```python
from build123d import *

# Parameters (mm, degrees)
CHANFREIN1_SIZE                                = 0.2
FRAISAGE_POUR_VIS_T_TE_FRAIS_E_M31_D           = 3.4
FRAISAGE_POUR_VIS_T_TE_FRAIS_E_M31_CSINK_D     = 6.3
FRAISAGE_POUR_VIS_T_TE_FRAIS_E_M31_CSINK_ANGLE = 90
CONG_1_R                                       = 2
FRAISAGE_POUR_VIS_T_TE_FRAIS_E_M22_D           = 2.2
FRAISAGE_POUR_VIS_T_TE_FRAIS_E_M22_CSINK_D     = 4.4
FRAISAGE_POUR_VIS_T_TE_FRAIS_E_M22_CSINK_ANGLE = 90


with BuildPart() as part:
    # Esquisse1 → Révolution1 (revolve)
    with BuildSketch(Plane(origin=(0, 0, 0), x_dir=(0, 0, -1), z_dir=(1, 0, 0))):
        Polygon((-5, -3), (-5, 0), (-8.5, 0), (-8.5, 6), (-18, 6), (-18, 3), (-11, 3), (-11, -3), align=None)
    revolve(axis=Axis((0, 0, 0), (0, -1, 0)))

    # Chanfrein1
    chanfrein1_edges = [part.edges().sort_by_distance(p)[0] for p in [
        (0, -3, -11),
    ]]
    chamfer(chanfrein1_edges, length=CHANFREIN1_SIZE)

    # Fraisage pour vis à tête fraisée M31 (through all)
    with Locations(Plane(origin=(0, 6, -13.5), x_dir=(0, 0, 1), z_dir=(0, 1, 0))):
        with Locations((0, 0), (20.25, 11.691342951), (20.25, -11.691342951)):
            CounterSinkHole(FRAISAGE_POUR_VIS_T_TE_FRAIS_E_M31_D / 2, FRAISAGE_POUR_VIS_T_TE_FRAIS_E_M31_CSINK_D / 2, counter_sink_angle=FRAISAGE_POUR_VIS_T_TE_FRAIS_E_M31_CSINK_ANGLE)

    # Congé1
    # the kernel refuses this fillet: 2 mm, written as the material it takes off along each edge
    with BuildSketch(Plane(origin=(0, 6, 0), x_dir=(0, 0, 1), z_dir=(1, 0, 0))) as cong_1_piece_1:
        with BuildLine():
            CenterArc((18 - CONG_1_R, CONG_1_R), CONG_1_R, 270, 90)
            Line((18, CONG_1_R), (18, 0))
            Line((18, 0), (18 - CONG_1_R, 0))
        make_face()
    revolve(axis=Axis((0, 6, 0), (0, -1, 0)), mode=Mode.SUBTRACT)

    # Fraisage pour vis à tête fraisée M22 (through all)
    with Locations(Plane(origin=(0, -3, 0), x_dir=(-1, 0, 0), z_dir=(0, -1, 0))):
        with Locations((0, 6.5), (-5.629165125, -3.25), (5.629165125, -3.25)):
            CounterSinkHole(FRAISAGE_POUR_VIS_T_TE_FRAIS_E_M22_D / 2, FRAISAGE_POUR_VIS_T_TE_FRAIS_E_M22_CSINK_D / 2, counter_sink_angle=FRAISAGE_POUR_VIS_T_TE_FRAIS_E_M22_CSINK_ANGLE)


solid = part.part
```
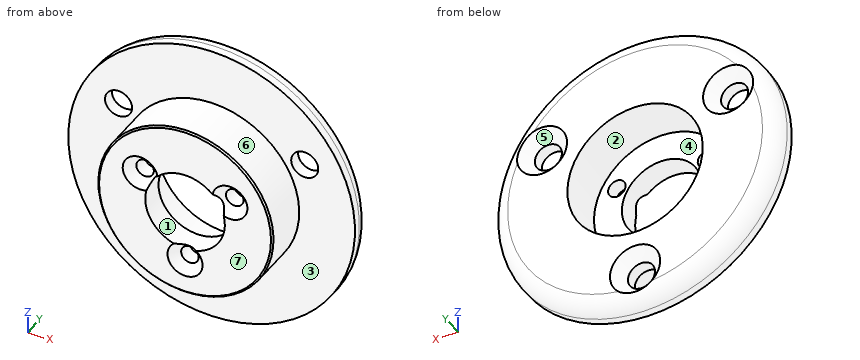
Input: part model. Units: mm. Frame: model coordinates. Face numbers are marked on the shaded views. A direction names the side the tool comes from. Coordinates: 2 decimals unless noted, no trailing zeros. Loops run counter-clockwise (first coordinate to the right, second up) from the corner with the lowest first, then second, coordinate; pieces in that order, holes last.
Q1. Section B-B, the plane x = 0. Give the number of separate pieces and of enclosed holes in the cut face, and give its area (3 significant figures).
Results are:
separate pieces: 4
enclosed holes: 0
area: 86.4 mm2
Q2. Contact query for flat-ended pins moving along their axis: pin 1 (2 mm diameter, centred on x = 5.63, z = 3.25, fed in from +Y); pin 2 (5.5 mm diameter, centred on x = -11.69, z = 6.75, fed in from +Y); pin 3 (2 mm diameter, centred on x = 9.5, z = 13, fed in from -Y); pin 4 (1 mm diameter, centred on x = 12, y = 3.5, fed in from +Z). Output: stop coordinate, or through.
Results are:
pin 1: passes through
pin 2: stops at y = 5.6
pin 3: stops at y = 3
pin 4: stops at z = 13.85
Q3. Section A-A, the plane z = 0. Return the cut outline in (x, y).
Results are:
outline: (-18, 3) - (-11, 3) - (-11, -2.8) - (-10.8, -3) - (-5, -3) - (-5, 0) - (-8.5, 0) - (-8.5, 6) - (-16, 6) arc R2 ccw to (-18, 4) - close; (5, -3) - (10.8, -3) - (11, -2.8) - (11, 3) - (18, 3) - (18, 4) arc R2 ccw to (16, 6) - (8.5, 6) - (8.5, 0) - (5, 0) - close
Q4. Line query: line 1 along X through (y, z) = (3.35, 6.75); line 2 along X through (y, z) = (-1, -1); line 3 along Z through (x, y) = (-4.5, -2.25). Output: solid intervals per line, ascending.
Results are:
line 1: x = -16.69 to -13.39, -9.99 to -5.17, 5.17 to 9.99, 13.39 to 16.69
line 2: x = -10.95 to -4.9, 4.9 to 10.95
line 3: z = -10.04 to -2.18, 2.18 to 2.34, 4.16 to 10.04
Q5. Mould query, pull axis X, two halves, no side actions, for the marked faces 4, 5, 6 and 7. Classes: +X half, -X half, draft (parallel to the pull), parting line (faces both ways), or undercut.
Results are:
face 4: undercut
face 5: undercut
face 6: parting line
face 7: draft
Q6. Set-up query: the marked faces 1, 2 and 3. Return all of +Z, -Z, +X, -X, +Y, -Y with unobstructed straight access to the full face (end or side cutting, diameter ignored); none if empty.
Results are:
face 1: +Y, -Y
face 2: +Y
face 3: -Y
